Part model, mm, in its own coordinate system. Face numbers are marked on the shaded views. A direction names the side the tool comes from. Give positions to 0.01 mm unless a question says otherwise; leave off trailing zeros. Order: outer loops, then holes, each group sorted by start corner. A loop starts at its lowest first (then second) coordinate and runs counter-clockwise, first axis right, second up. Notation, with made-up numbers: M 72,-16.75 L 79,-16.75 A14 cw 79,7.25 Z; hole C 73.5,29.5 d1. An arc over 180 degrees is marked long. Return JSON: item names as keys, results as strings.
from build123d import *

# Parameters (mm, degrees)
BOSS_EXTRUDE1_DEPTH = 5.81


with BuildPart() as part:
    # Sketch2 → Boss-Extrude1 (new body)
    with BuildSketch(Plane.XY):
        Polygon((0, 29.95), (0, 14.975), (0, 0), (68.15, 0), (68.15, 14.975), (68.15, 29.95), align=None)
        with BuildLine():
            ThreePointArc((11.86, 10.7), (8.83711851, 11.95211851), (7.585, 14.975))
            ThreePointArc((7.585, 14.975), (8.83711851, 17.99788149), (11.86, 19.25))
            Line((11.86, 19.25), (20.035, 19.25))
            Line((20.035, 19.25), (28.215, 19.25))
            ThreePointArc((28.215, 19.25), (31.23788149, 17.99788149), (32.49, 14.975))
            ThreePointArc((32.49, 14.975), (31.23788149, 11.95211851), (28.215, 10.7))
            Line((28.215, 10.7), (20.035, 10.7))
            Line((20.035, 10.7), (11.86, 10.7))
        make_face(mode=Mode.SUBTRACT)
        with BuildLine():
            add(Edge.make_bspline(
                [(57.755, 22.155), (60.54, 18.565), (60.54, 14.975)],
                knots=[0, 0, 0, 0.5, 0.5, 0.5], degree=2))
            add(Edge.make_bspline(
                [(60.54, 14.975), (60.54, 11.385), (57.755, 7.795)],
                knots=[0.5, 0.5, 0.5, 1, 1, 1], degree=2))
            Line((57.755, 7.795), (50.395, 7.795))
            Line((50.395, 7.795), (43.035, 7.795))
            add(Edge.make_bspline(
                [(43.035, 7.795), (40.25, 11.385), (40.25, 14.975)],
                knots=[0, 0, 0, 0.5, 0.5, 0.5], degree=2))
            add(Edge.make_bspline(
                [(40.25, 14.975), (40.25, 18.565), (43.035, 22.155)],
                knots=[0.5, 0.5, 0.5, 1, 1, 1], degree=2))
            Line((43.035, 22.155), (50.395, 22.155))
            Line((50.395, 22.155), (57.755, 22.155))
        make_face(mode=Mode.SUBTRACT)
    extrude(amount=BOSS_EXTRUDE1_DEPTH)


solid = part.part
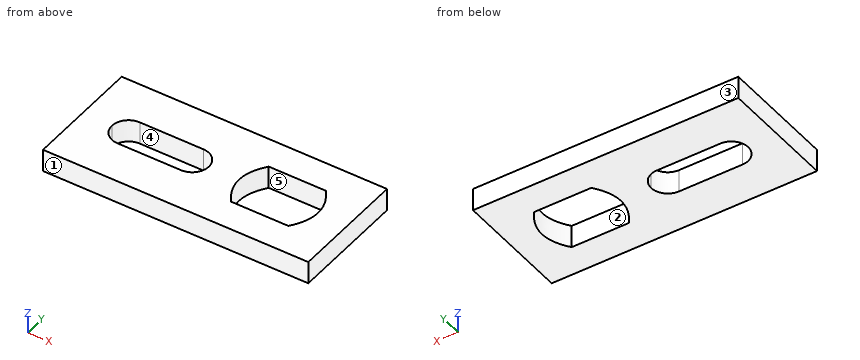
Q1. Band-saw the part on B-B (z = 3.05). Give the number of separate pieces and of enclosed holes in the cut face, then the cut area to 3 significant figures.
Established:
{"separate pieces": "1", "enclosed holes": "2", "area": "1,580 mm²"}
Q2. Band-saw the part on C-C (x = 51). Give the cut face in (y, z) (3 decimals), then the cut area to 3 significant figures.
Established:
{"outline": "M 0,0 L 7.795,0 L 7.795,5.81 L 0,5.81 Z; M 22.155,0 L 29.95,0 L 29.95,5.81 L 22.155,5.81 Z", "area": "90.6 mm²"}
Q3. Band-saw the part on A-A (x = 15). Give the cut face in (y, z).
Established:
{"outline": "M 0,0 L 10.7,0 L 10.7,5.81 L 0,5.81 Z; M 19.25,0 L 29.95,0 L 29.95,5.81 L 19.25,5.81 Z"}
Q4. Two-plate mould, pull along X, no slides. Class the marked faces 3, 4 and 5: +X half, -X half, draft (parallel to the pull), parting line (faces both ways), or undercut.
Established:
{"face 3": "draft", "face 4": "undercut", "face 5": "undercut"}
Q5. Probe line 1 along Y through (x, z) = (26, 0.55); line 2 along Y through (x, z) = (48, 2.05) (3 decimals); line 3 along X through (y, z) = (16.25, 3.75). List the from-to ranges inside material, lowest first.
Established:
{"line 1": "y = 0 to 10.7, 19.25 to 29.95", "line 2": "y = 0 to 7.795, 22.155 to 29.95", "line 3": "x = 0 to 7.78, 32.3 to 40.34, 60.45 to 68.15"}
Q6. 3-axis set-ups, long thin cutter, end or side, ignore diameter. For the marked faces 1 and 2: which of +Z, -Z, +X, -X, +Y, -Y reach the whole face in a straight line?
Established:
{"face 1": "+Z, -Z, +X, -X, -Y", "face 2": "+Z, -Z"}
